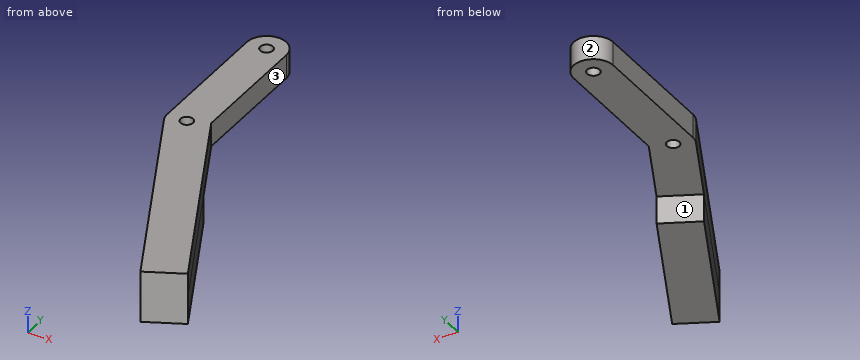
```python
from build123d import *

# Parameters (mm, degrees)
SALIENTE_EXTRUIR1_DEPTH = 6
CROQUIS2_R              = 1.6
CORTAR_EXTRUIR1_DEPTH   = 65.918146911
SALIENTE_EXTRUIR2_DEPTH = 7


with BuildPart() as part:
    # Croquis1 → Saliente-Extruir1 (new body)
    with BuildSketch(Plane.XY):
        with BuildLine():
            Line((-5, 33.48), (-5, 0))
            ThreePointArc((-5, 0), (0, -5), (5, 0))
            Line((5, 0), (5, 33.48))
            ThreePointArc((5, 33.48), (0, 38.48), (-5, 33.48))
        make_face()
        with BuildLine():
            ThreePointArc((5, 0), (1.357892891, -4.812081348), (-4.262450759, -2.613716421))
            Line((-4.262450759, -2.613716421), (22.256084979, -56.435340907))
            Line((22.256084979, -56.435340907), (31.518535738, -51.871624486))
            Line((31.518535738, -51.871624486), (5, 1.95))
            Line((5, 1.95), (5, 0))
        make_face()
    extrude(amount=SALIENTE_EXTRUIR1_DEPTH)

    # Croquis2 → Cortar-Extruir1 (cut, through all)
    with BuildSketch(Plane.XY.offset(6)):
        with Locations((0, 33.48)):
            Circle(CROQUIS2_R)
        Circle(CROQUIS2_R)
    extrude(amount=-CORTAR_EXTRUIR1_DEPTH, mode=Mode.SUBTRACT)

    # Croquis3 → Saliente-Extruir2 (add)
    with BuildSketch(Plane(origin=(0, 0, 0), x_dir=(-1, 0, 0), z_dir=(0, 0, -1))):
        Polygon((-31.518535738, -51.871624486), (-22.256084979, -56.435340907), (-4.577061154, -20.554257916), (-13.839511913, -15.990541495), align=None)
    extrude(amount=SALIENTE_EXTRUIR2_DEPTH)


solid = part.part
```
Can you work these out from the model? Positions are in its coordinate system, mm. Face numbers are marked on the shaded views. A direction names the side the tool comes from. Give positions to 0.01 mm unless a question says otherwise; leave off trailing zeros. Loops run counter-clockwise (first coordinate to the right, second up) from the corner with the lowest first, then second, coordinate; pieces in that order, holes last. Notation, with made-up numbers: M 62.25,-35 L 116.25,-35 A19 cw 116.25,-17 Z; hole C 0.5,80 d8. An arc over 180 degrees is marked long. Answer in a Markdown table with one row per item.
1. If I drill on line 1 along Y through (x, z) = (0, 4.65); line 2 along Z through (x, y) = (-2, 28); line 3 along X through (y, z) = (8, 0.75), over which ranges is the centre line in solid material (lowest first)?
Taken from the geometry:
| item | result |
|---|---|
| line 1 | y = -11.26 to -1.6, 1.6 to 31.88, 35.08 to 38.48 |
| line 2 | z = 0 to 6 |
| line 3 | x = -5 to 5 |
2. Suppose I cut it at B-B on x = 0. Write out the boundary of the cut face in (y, z), plus the area to 3 significant figures.
Taken from the geometry:
| item | result |
|---|---|
| outline | M -11.26,0 L -1.6,0 L -1.6,6 L -11.26,6 Z; M 1.6,0 L 31.88,0 L 31.88,6 L 1.6,6 Z; M 35.08,0 L 38.48,0 L 38.48,6 L 35.08,6 Z |
| area | 260 mm² |
3. Suppose I cut it at A-A on z = 4. Write out the boundary of the cut face in (x, y), plus the area to 3 significant figures.
Taken from the geometry:
| item | result |
|---|---|
| outline | M -5,0 A5 ccw -4.26,-2.61 L 22.26,-56.44 L 31.52,-51.87 L 5,1.95 L 5,33.48 A5 ccw -5,33.48 Z; hole C 0,0 d3.2; hole C 0,33.48 d3.2 |
| area | 982 mm² |
4. For pin 1 Ø4 at (x, z) = (14.5, 1.5) entering from +Y; pin 2 Ø20.5 at (x, y) = (2, 19) entering from -Z; pin 3 Ø2 at (x, z) = (8.5, 2.5) entering from -Y, each with a flat end and sliding along its axis, tell me the tip position at first contact or that it passes through.
Taken from the geometry:
| item | result |
|---|---|
| pin 1 | stops at y = -13.27 |
| pin 2 | stops at z = 0 |
| pin 3 | stops at y = -30.55 |
5. Suppose I cut it at C-C on y = 26.5. Write out the boundary of the cut face in (x, z), plus the area to 3 significant figures.
Taken from the geometry:
| item | result |
|---|---|
| outline | M -5,0 L 5,0 L 5,6 L -5,6 Z |
| area | 60.0 mm² |
6. Suppose I cut it at D-D on x = 7. Write out the boundary of the cut face in (y, z), plus the area to 3 significant figures.
Taken from the geometry:
| item | result |
|---|---|
| outline | M -25.47,-7 L -19.36,-7 L -19.36,0 L -2.11,0 L -2.11,6 L -25.47,6 Z |
| area | 183 mm² |
7. Which directions (+Z, -Z, +X, -X, +Y, -Y) give clear straight access to the entire face, cutting with the end or side of a thin tool? Please do the marked faces 1, 2 and 3.
Taken from the geometry:
| item | result |
|---|---|
| face 1 | -Z, -X, +Y |
| face 2 | +Z, -Z, +Y |
| face 3 | +Z, -Z, +X, +Y |
